Geometry check sheet. Reference: the model listing, model coordinates, mm. A direction names the side the tool comes from. Round coordinates to 2 decimals unless told otherwise and drop trailing zeros. Order: outer loops, then holes, each group sorted by start corner. A loop starts at its lowest first (then second) coordinate and runs counter-clockwise, first axis right, second up.
(1) Cross-section at A-A on x = 0. Enter the section's corners in (y, z) (3 decimals).
(2) Cross-section at B-B on z = 46.5. Enter the section's corners in (x, y), and give its area (3 significant figures).
(3) Draft check along Y on faces 1 (the face through (26.2, -26.1, 38.5)), 2 (the face through (23.386, -23.674, 66.59)), 3 (the face through (0, 0, 0)). Enter one of: pulls with the +Y half, pulls with the -Y half, needs draft (parallel to the pull), parting line crosses it, or undercut.
(4) Set-up check for faces 4 (the face through (-23.1, -24.71, 71.54)), 5 (the face through (28.65, 0, 37)): record each of +Z, -Z, +X, -X, +Y, -Y from which the full face is reachable in a straight line by a thin tool's end or side.
(5) Cross-section at D-D on y = -7.5. Enter the section's corners in (x, z), and give its area (3 significant figures).
(6) Gauge pin test, flat ends, axial feed: P1, Ø4, axis at x = 23.575, y = -23.575, coming from the +Z side; P2, Ø12, axis at x = -4.5, y = 16.5, coming from the +Z side; P3, Ø2, axis at x = 23.575, y = 23.575, coming from the +Z side. Record the tip position at first contact, or that the pin passes through.
(7) Thickness scan on L1, parallel to Z at x = 8, y = -20; L2, parallel to Z at x = -7, y = 14.5; L3, parallel to X at y = 1, z = 83. Record the ranges inside material, lowest first.
Autodesk Inventor part; units mm, degrees
ref_plane "YZ Plane" through (0, 0, 0) normal (1, 0, 0) x (0, 1, 0)
ref_plane "XZ Plane" through (0, 0, 0) normal (0, 1, 0) x (-1, 0, 0)
ref_plane "XY Plane" through (0, 0, 0) normal (0, 0, 1) x (1, 0, 0)
sketch "Skizze1" plane through (0, 0, 0) normal (0, 0, 1) x (1, 0, 0)
  line L0 (-40.11, 0) -> (40.11, 0)
  line L1 (0, -40.11) -> (0, 40.11)
  line L2 (28.65, -28.65) -> (-28.65, -28.65)
  line L3 (-28.65, -28.65) -> (-28.65, 28.65)
  line L4 (-28.65, 28.65) -> (28.65, 28.65)
  line L5 (28.65, 28.65) -> (28.65, -28.65)
  line L6 (28.65, -28.65) -> (-28.65, 28.65) construction
  line L7 (-28.65, -28.65) -> (28.65, 28.65) construction
  point P0 (0, 0)
  dimension "d0" = 57.3
  dimension "d1" = 57.3
extrude "Extrusion1" add sketch "Skizze1" along normal blind 76
sketch "Skizze2" plane through (0, 0, 76) normal (0, 0, 1) x (1, 0, 0)
  circle A0 centre (0, 0) radius 19
  dimension "d4" = 38
extrude "Extrusion2" add sketch "Skizze2" along normal blind 1.6
sketch "Skizze3" plane through (0, 0, 77.6) normal (0, 0, 1) x (1, 0, 0)
  circle A0 centre (0, 0) radius 3.175
  dimension "d7" = 6.35
extrude "Extrusion3" add sketch "Skizze3" along normal blind 22
sketch "Skizze4" plane through (0, 0, 76) normal (0, 0, 1) x (1, 0, 0)
  circle A0 centre (0, 0) radius 19
  line L0 (28.65, 28.65) -> (-28.65, 28.65)
  line L1 (-28.65, 28.65) -> (-28.65, -28.65)
  line L2 (-28.65, -28.65) -> (28.65, -28.65)
  line L3 (28.65, -28.65) -> (28.65, 28.65)
  line L4 (23.575, -23.575) -> (-23.575, -23.575)
  line L5 (-23.575, -23.575) -> (-23.575, 23.575)
  line L6 (-23.575, 23.575) -> (23.575, 23.575)
  line L7 (23.575, 23.575) -> (23.575, -23.575)
  line L8 (23.575, -23.575) -> (-23.575, 23.575) construction
  line L9 (-23.575, -23.575) -> (23.575, 23.575) construction
  dimension "d10" = 47.15
  dimension "d11" = 47.15
hole "Bohrung1" at (-23.575, 23.575, 76) at (23.575, 23.575, 76) at (23.575, -23.575, 76) at (-23.575, -23.575, 76) direction (0, 0, -1) diameter 2.459 depth 8.8 tip angle 118
chamfer "Fasen1" distance 5 angle 45 4 edges at (28.65, -28.65, 38) (28.65, 28.65, 38) (-28.65, 28.65, 38) (-28.65, -28.65, 38)
equation "\"d1\" = d0"
equation "\"d11\" = d10"
properties part number "Motor ST nema 23"
Found:
1. outline: (-28.65, 0) - (28.65, 0) - (28.65, 76) - (19, 76) - (19, 77.6) - (3.175, 77.6) - (3.175, 99.6) - (-3.175, 99.6) - (-3.175, 77.6) - (-19, 77.6) - (-19, 76) - (-28.65, 76) - close
2. outline: (-28.65, -23.65) - (-23.65, -28.65) - (23.65, -28.65) - (28.65, -23.65) - (28.65, 23.65) - (23.65, 28.65) - (-23.65, 28.65) - (-28.65, 23.65) - close
2. area: 3,230 mm2
3. face 1: pulls with the -Y half
3. face 2: undercut
3. face 3: needs draft
4. face 4: +Z
4. face 5: +Z, -Z, +X, +Y, -Y
5. outline: (-28.65, 0) - (28.65, 0) - (28.65, 76) - (17.46, 76) - (17.46, 77.6) - (-17.46, 77.6) - (-17.46, 76) - (-28.65, 76) - close
5. area: 4,410 mm2
6. P1: stops at z = 76
6. P2: stops at z = 77.6
6. P3: stops at z = 67.06
7. L1: z = 0 to 76
7. L2: z = 0 to 77.6
7. L3: x = -3.01 to 3.01
